Verification items for the finished model (mm, model axes). A direction names the side the tool comes from. Round coordinates to 2 decimals unless told otherwise and drop trailing zeros. Write each question's results on one line, items separated by ' | '.
from build123d import *

# Parameters (mm, degrees)
BOSS_EXTRUDE1_DEPTH = 10
FILLET1_R           = 2
SKETCH3_R           = 1.9
CUT_EXTRUDE3_DEPTH  = 240
CUT_EXTRUDE4_DEPTH  = 5
SKETCH6_R           = 1.75
CUT_EXTRUDE8_DEPTH  = 10
SKETCH7_R           = 23.25
SKETCH7_R_2         = 21
BOSS_EXTRUDE2_DEPTH = 7
CUT_EXTRUDE9_DEPTH  = 5
SKETCH9_R           = 1.75
CUT_EXTRUDE10_DEPTH = 10


with BuildPart() as part:
    # Sketch1 → Boss-Extrude1 (new body)
    with BuildSketch(Plane.XY):
        with BuildLine():
            Line((-192.723621419, -64.866060055), (-18.311266157, 32.725334708))
            ThreePointArc((-18.311266157, 32.725334708), (33.388989093, 17.071186467), (15.807091975, -34.005673693))
            Line((15.807091975, -34.005673693), (-165.428934914, -118.250866776))
            ThreePointArc((-165.428934914, -118.250866776), (-204.785799768, -104.703276995), (-192.723621419, -64.866060055))
        make_face()
    extrude(amount=BOSS_EXTRUDE1_DEPTH)

    # Fillet1
    fillet1_edges = [part.edges().sort_by_distance(p)[0] for p in [
        (33.388989093, 17.071186467, 10),
        (-105.517443788, -16.070362674, 10),
        (-204.785799768, -104.703276995, 10),
        (-105.517443788, -16.070362674, 0),
        (33.388989093, 17.071186467, 0),
        (-74.81092147, -76.128270234, 0),
        (-204.785799768, -104.703276995, 0),
        (-74.81092147, -76.128270234, 10),
    ]]
    fillet(fillet1_edges, radius=FILLET1_R)

    # Sketch3 → Cut-Extrude3 (cut)
    with BuildSketch(Plane.XY.offset(10)):
        with Locations((-178.074608494, -91.046327822)):
            Circle(SKETCH3_R)
    extrude(amount=-CUT_EXTRUDE3_DEPTH, mode=Mode.SUBTRACT)

    # Sketch4 → Cut-Extrude4 (cut)
    with BuildSketch(Plane.XY.offset(10)):
        Polygon((1.949051074, -23.338757463), (-0.99159812, -25.380566053), (-0.693664608, -28.948147254), (2.544918098, -30.473919864), (5.485567292, -28.432111274), (5.18763378, -24.864530073), align=None)
        Polygon((19.237431318, 13.357306475), (22.476014024, 11.831533865), (25.416663218, 13.873342455), (25.118729706, 17.440923655), (21.880147001, 18.966696266), (18.939497807, 16.924887676), align=None)
        Polygon((-21.186482393, 9.981450988), (-21.484415905, 13.549032188), (-24.72299861, 15.074804799), (-27.663647804, 13.032996209), (-27.365714292, 9.465415008), (-24.127131587, 7.939642398), align=None)
    extrude(amount=-CUT_EXTRUDE4_DEPTH, mode=Mode.SUBTRACT)

    # Sketch6 → Cut-Extrude8 (cut)
    with BuildSketch(Plane.XY.offset(10)):
        with Locations((2.246984586, -26.906338663)):
            Circle(SKETCH6_R)
        with Locations((-24.425065098, 11.507223598)):
            Circle(SKETCH6_R)
        with Locations((22.178080512, 15.399115065)):
            Circle(SKETCH6_R)
    extrude(amount=-CUT_EXTRUDE8_DEPTH, mode=Mode.SUBTRACT)

    # Sketch7 → Boss-Extrude2 (add)
    with BuildSketch(Plane.XY.offset(10)):
        Circle(SKETCH7_R)
        Circle(SKETCH7_R_2, mode=Mode.SUBTRACT)
    extrude(amount=BOSS_EXTRUDE2_DEPTH)

    # Sketch8 → Cut-Extrude9 (cut)
    with BuildSketch(Plane(origin=(0, 0, 0), x_dir=(-1, 0, 0), z_dir=(0, 0, -1))):
        Polygon((181.262166534, -92.676012988), (181.079736268, -89.100664166), (177.892178228, -87.470979), (174.887050454, -89.416642655), (175.06948072, -92.991991477), (178.25703876, -94.621676643), align=None)
    extrude(amount=-CUT_EXTRUDE9_DEPTH, mode=Mode.SUBTRACT)

    # Sketch9 → Cut-Extrude10 (cut)
    with BuildSketch(Plane.XY.offset(10)):
        Circle(SKETCH9_R)
    extrude(amount=-CUT_EXTRUDE10_DEPTH, mode=Mode.SUBTRACT)


solid = part.part
1) Draft check along X on faces 1 (the cylindrical face through (-76.32, -76.2, 0.6)), 2 (the cylindrical face through (22.176, 6.984, 13.451)), 3 (the cylindrical face through (20.03, 6.31, 13.45)). Enter one of: pulls with the +X half, pulls with the -X half, needs draft (parallel to the pull), parting line crosses it, or undercut.
Calculated:
face 1: pulls with the +X half | face 2: parting line crosses it | face 3: undercut
2) Access from +Z, -Z, +X, -X, +Y, -Y to the whole of each face (thin tool, end or side, straight path). Record for faces 4 (the flat face through (0, -4, 10)), 5 (the cylindrical face through (-76.32, -76.2, 9.4)), 6 (the flat face through (-179, -93, 5)).
Calculated:
face 4: +Z | face 5: +Z, +X, -Y | face 6: -Z
3) Depth check by flat-ended pin: P1, Ø4, axis at x = 2.25, y = -26.91, coming from the +Z side; P2, Ø5, axis at x = -179.5, y = -90.5, coming from the -Z side; P3, Ø12.5, axis at x = 1, y = -6.5, coming from the +Z side; P4, Ø5, axis at y = -47.5, z = 4.5, coming from the -X side. Enter the tip coordinate at first touch or a pass-through.
Calculated:
P1: stops at z = 5 | P2: stops at z = 0 | P3: stops at z = 10 | P4: stops at x = -166.16
4) Material ranges on line 1 (Y direction, x = 0, z = 12.25); line 2 (Y direction, x = 0, z = 4.5); line 3 (Z direction, x = -59.5, y = 3), recorded low to high. Write a range as [from, to].
Calculated:
line 1: y = [-23.25, -21], [21, 23.25] | line 2: y = [-41.35, -1.75], [1.75, 37.5] | line 3: z = [0, 10]
